For this review, use the dimensioned drawing (mm, ordinates from the lowest corner) and the shaded views. A direction names the side the tool comes from. Coordinates: 2 decimals unless noted, no trailing zeros. Order: outer loops, then holes, each group sorted by start corner. A loop starts at its lowest first (then second) coordinate and runs counter-clockwise, first axis right, second up. Notation, with made-up numbers: M 24,-35 L 57,-35 A13 cw 57,-28 Z; hole C -20,56.5 d1. An arc over 180 degrees is marked long. Use CSV: the item, a comma, the result in double quotes.
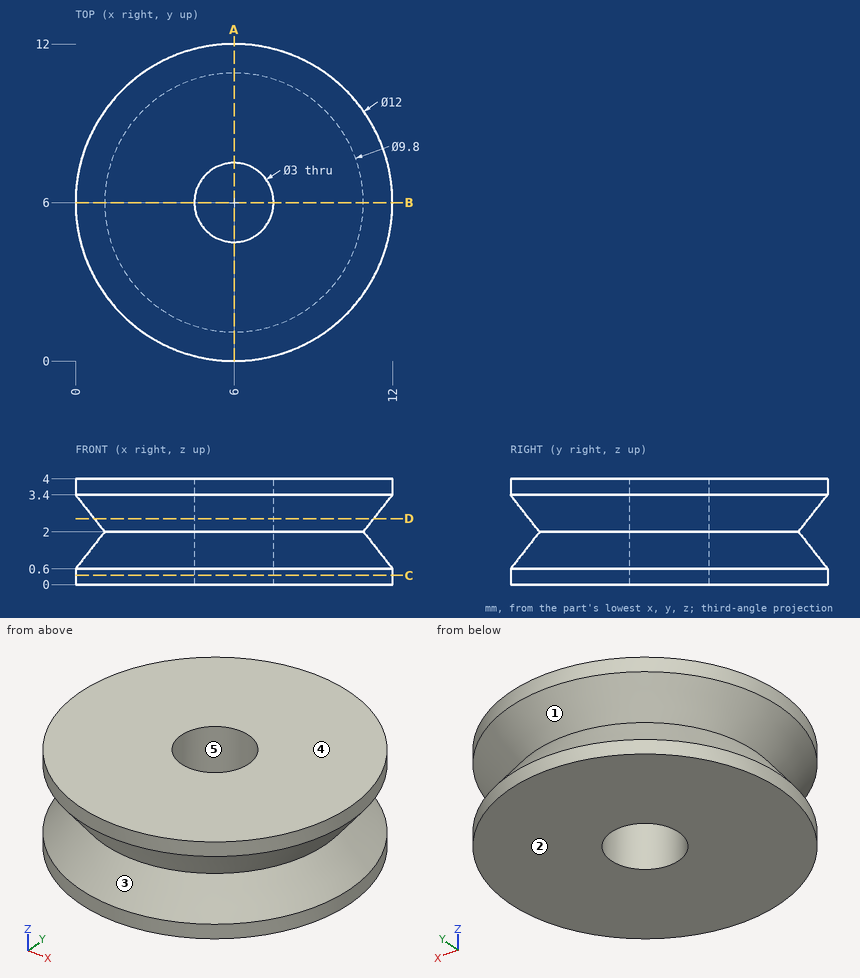
Item 1: Add section A-A on x = 6. State the section outline as (y, z) points.
Solutions:
outline,"M 0,0 L 4.5,0 L 4.5,4 L 0,4 L 0,3.4 L 1.1,2 L 0,0.6 Z; M 7.5,0 L 12,0 L 12,0.6 L 10.9,2 L 12,3.4 L 12,4 L 7.5,4 Z"
Item 2: To check wall thickness, follow line 1 along Y through (x, z) = (7.25, 3.15); line 2 along Y through (x, z) = (6, 1.25); line 3 along X through (y, z) = (6.5, 3.35). State the ranges of each line that lie inside material, in increasing order. Write a range as [from, to].
Solutions:
line 1,"[0.33, 5.17], [6.83, 11.67]"
line 2,"[0.51, 4.5], [7.5, 11.49]"
line 3,"[0.06, 4.59], [7.41, 11.94]"
Item 3: For the marked faces 1 and 2, list the 3-axis set-ups (+Z, -Z, +X, -X, +Y, -Y) from which the entire face can be reached by the end or side of a thin tool; tool diameter is ignored.
Solutions:
face 1,"none"
face 2,"-Z, +X, -X, +Y, -Y"
Item 4: Draft analysis for pull direction Y (two halves, no side actions). For the marked faces 3, 4 and 5, state which applies: released by +Y, released by -Y, zero draft, split by the parting line, or undercut.
Solutions:
face 3,"split by the parting line"
face 4,"zero draft"
face 5,"undercut"
Item 5: Add section C-C on z = 0.35. State the section outline as (x, y) points, and give its area (3 significant figures).
Solutions:
outline,"C 6,6 d12; hole C 6,6 d3"
area,"106 mm^2"
Item 6: Add section D-D on z = 2.5. State the section outline as (x, y) points.
Solutions:
outline,"C 6,6 d10.59; hole C 6,6 d3"
Item 7: Clearance check with flat-ended pins moving along their axes: pin 1 Ø1 at (x, z) = (9.5, 1) entering from -Y; pin 2 Ø2 at (x, z) = (8.5, 3) entering from +Y; pin 3 Ø2 at (y, z) = (4.5, 0.5) entering from +X. State where each tip first meets the part, or that it passes through.
Solutions:
pin 1,"y = 0.92"
pin 2,"y = 11.79"
pin 3,"x = 11.98"
